from build123d import *

# Parameters (mm, degrees)
SKETCH1_R           = 12
BOSS_EXTRUDE1_DEPTH = 4
SKETCH7_W           = 10
SKETCH7_H           = 7
SKETCH7_R           = 2
BOSS_EXTRUDE4_DEPTH = 4
SKETCH8_R           = 20
CUT_EXTRUDE3_DEPTH  = 86.850160163
CUT_EXTRUDE4_DEPTH  = 87.407464955


with BuildPart() as part:
    # Sketch1 → Boss-Extrude1 (new body)
    with BuildSketch(Plane(origin=(0, 0, 0), x_dir=(0, 0, -1), z_dir=(1, 0, 0))):
        with BuildLine():
            Line((62.5, 58), (-4.5, 58))
            ThreePointArc((-4.5, 58), (-62.5, 0), (-4.5, -58))
            Line((-4.5, -58), (62.5, -58))
            Line((62.5, -58), (62.5, 58))
        make_face()
        with Locations((-4.5, 0)):
            Circle(SKETCH1_R, mode=Mode.SUBTRACT)
    extrude(amount=BOSS_EXTRUDE1_DEPTH)

    # Sketch7 → Boss-Extrude4 (add)
    # profile 1 of 2: a face of its own
    with BuildSketch(Plane(origin=(0, 0, -62.5), x_dir=(-1, 0, 0), z_dir=(0, 0, -1))):
        with Locations((5, 54.5)):
            Rectangle(SKETCH7_W, SKETCH7_H)
        with Locations((5, 54.5)):
            Circle(SKETCH7_R, mode=Mode.SUBTRACT)
    # profile 2 of 2: a face of its own
    with BuildSketch(Plane(origin=(0, 0, -62.5), x_dir=(-1, 0, 0), z_dir=(0, 0, -1))):
        with Locations((5, -54.5)):
            Rectangle(SKETCH7_W, SKETCH7_H)
        with Locations(Location((5, -54.5, 0), (0, 0, 180))):
            Circle(SKETCH7_R, mode=Mode.SUBTRACT)
    extrude(amount=-BOSS_EXTRUDE4_DEPTH)

    # Sketch8 → Cut-Extrude3 (cut, through all)
    with BuildSketch(Plane.ZY):
        with Locations((4.5, 0)):
            Circle(SKETCH8_R)
    extrude(amount=-CUT_EXTRUDE3_DEPTH, mode=Mode.SUBTRACT)

    # Sketch9 → Cut-Extrude4 (cut, through all)
    with BuildSketch(Plane(origin=(4, 0, 0), x_dir=(0, 0, -1), z_dir=(1, 0, 0))):
        with BuildLine():
            Line((-46.5, 40), (-46.5, -40))
            ThreePointArc((-46.5, -40), (-62.5, 0), (-46.5, 40))
        make_face()
    extrude(amount=-CUT_EXTRUDE4_DEPTH, mode=Mode.SUBTRACT)


solid = part.part
Can you work these out from the model? Positions are in its coordinate system, mm. A direction names the side the tool comes from. Coordinates: 2 decimals unless noted, no trailing zeros. Write each loop counter-clockwise with the first axis right and the second up, starting at its lowest first coordinate (ties: lowest second). Pieces come first, ordered by that corner, then holes.
Q1. Imagine slicing it at A-A, the plane x = -5. List the corners of the cut face in (y, z) for me, plus the area to 3 significant figures.
Results found:
outline: (-58, -62.5) - (-56.5, -62.5) - (-56.5, -58.5) - (-58, -58.5) - close; (-52.5, -62.5) - (-51, -62.5) - (-51, -58.5) - (-52.5, -58.5) - close; (51, -62.5) - (52.5, -62.5) - (52.5, -58.5) - (51, -58.5) - close; (56.5, -62.5) - (58, -62.5) - (58, -58.5) - (56.5, -58.5) - close
area: 24.0 mm2
Q2. Imagine slicing it at B-B, the plane y = 0. List the corners of the cut face in (x, z) for me.
Results found:
outline: (0, -62.5) - (4, -62.5) - (4, -15.5) - (0, -15.5) - close; (0, 24.5) - (4, 24.5) - (4, 46.5) - (0, 46.5) - close
Q3. Please list where these lines run through material, in increasing order: L1, parallel to Y at x = -5, z = -60.7; L2, parallel to Y at x = 2.8, z = 4.5; L3, parallel to X at y = -54.5, z = -61.65.
Results found:
L1: y = -58 to -56.5, -52.5 to -51, 51 to 52.5, 56.5 to 58
L2: y = -58 to -20, 20 to 58
L3: x = -10 to -7, -3 to 4
Q4. For P1, Ø4, axis at x = 0.5, z = 10.5, coming from the -Y side; P2, Ø3.5, axis at x = -5, y = 53.5, coming from the +Z side; P3, Ø8, axis at y = -30, z = -16, coming from the -X side, each with a flat end and sliding along its axis, tell me the tip position at first contact or that it passes through.
Results found:
P1: stops at y = -57.86
P2: stops at z = -58.5
P3: stops at x = 0
Q5. Imagine slicing it at D-D, the plane x = 2.5. List the corners of the cut face in (y, z) for me.
Results found:
outline: (-58, -62.5) - (58, -62.5) - (58, 4.5) arc R58 ccw to (40, 46.5) - (-40, 46.5) arc R58 ccw to (-58, 4.5) - close; hole circle Ø40 at (0, 4.5)
Q6. Imagine slicing it at C-C, the plane z = 13.5. List the corners of the cut face in (x, y) for me.
Results found:
outline: (0, -57.3) - (4, -57.3) - (4, -17.86) - (0, -17.86) - close; (0, 17.86) - (4, 17.86) - (4, 57.3) - (0, 57.3) - close
Q7. If we mould it in two halves opening along X, with no side actions, what happens to faces 4 (the face through (-4.74, 56.483, -60.528)), 5 (the face through (-5.26, -56.483, -60.528)), 6 (the face through (-5, -51, -61)), 7 (the face through (-10, 54, -61))? For each: +X half, -X half, draft (parallel to the pull), parting line (faces both ways), or undercut.
Results found:
face 4: undercut
face 5: undercut
face 6: draft
face 7: -X half
Q8. Which directions (+Z, -Z, +X, -X, +Y, -Y) give clear straight access to the entire face, cutting with the end or side of a thin tool? Please do faces 1 (the face through (0.2, 13.7, -62.5)), 2 (the face through (-7.2, 54.5, -58.5)), 3 (the face through (-5, 51, -61)).
Results found:
face 1: -Z, +X, -X, +Y, -Y
face 2: +Z, -X, +Y, -Y
face 3: +Z, -Z, -X
